from build123d import *

# Parameters (mm, degrees)
F0_R     = 2.25
F0_R_2   = 15.5
F0_R_3   = 13
F1_DEPTH = 15
F2_DEPTH = 3
F3_W     = 12.2
F3_H     = 17.6
F4_DEPTH = 11.3
F5_R     = 1
F6_R     = 3


# Not quite as in the source:
# - ends of sketch curves that miss each other by under 0.0002 mm in the source are joined


with BuildPart() as f1:
    # F0 (on Front) → F1 (new body)
    with BuildSketch(Plane.XZ):
        with BuildLine():
            Line((-0.05, 27.5966813602), (-25.4, 27.5966813602))
            Line((-25.4, 27.5966813602), (-25.4, 7.5966813602))
            Line((-25.4, 7.5966813602), (-21.614542231, 7.5966813602))
            ThreePointArc((-21.614542231, 7.5966813602), (-23.4006244197, -4.2813010605), (-17.918619958, -14.9688724896))
            Line((-17.918619958, -14.9688724896), (-20.4748737342, -17.5251262658))
            ThreePointArc((-20.4748737342, -17.5251262658), (-20.4748737342, -22.4748737342), (-15.5251262658, -22.4748737342))
            Line((-15.5251262658, -22.4748737342), (-13.153804753, -20.1035522213))
            ThreePointArc((-13.153804753, -20.1035522213), (19.3130689129, -14.8757459996), (19.9528476572, 18.0031001889))
            Line((19.9528476572, 18.0031001889), (22.4748737342, 20.5251262658))
            ThreePointArc((22.4748737342, 20.5251262658), (22.4748737342, 25.4748737342), (17.5251262658, 25.4748737342))
            Line((17.5251262658, 25.4748737342), (14.8648475796, 22.8145950479))
            ThreePointArc((14.8648475796, 22.8145950479), (7.8051661925, 26.3642746914), (-9.5e-08, 27.5966326274))
            Line((-9.5e-08, 27.5966326274), (-0.05, 27.5966813602))
        make_face()
        with Locations((-18, -20)):
            Circle(F0_R, mode=Mode.SUBTRACT)
        Circle(F0_R_2, mode=Mode.SUBTRACT)
        with Locations((20, 23)):
            Circle(F0_R, mode=Mode.SUBTRACT)
        Circle(F0_R_2)
        Circle(F0_R_3, mode=Mode.SUBTRACT)
        Circle(F0_R_3)
    extrude(amount=-F1_DEPTH)

    # F0 (on Front) → F2 (cut)
    with BuildSketch(Plane.XZ):
        Circle(F0_R_2)
        Circle(F0_R_3, mode=Mode.SUBTRACT)
    extrude(amount=-F2_DEPTH, mode=Mode.SUBTRACT)

    # F3 (on face) → F4 (cut)
    with BuildSketch(Plane(origin=(-25.4, 0, 0), x_dir=(0, -1, 0), z_dir=(-1, 0, 0))):
        with Locations((-7.1, 17.5966813602)):
            Rectangle(F3_W, F3_H)
    extrude(amount=-F4_DEPTH, mode=Mode.SUBTRACT)

    # F5
    f5_edges = [f1.edges().sort_by_distance(p)[0] for p in [
        (-21.614542, 7.5, 7.596681),
    ]]
    fillet(f5_edges, radius=F5_R)

    # F6
    f6_edges = [f1.edges().sort_by_distance(p)[0] for p in [
        (-17.91862, 7.5, -14.968872),
        (-13.153805, 7.5, -20.103552),
        (19.952848, 7.5, 18.0031),
        (14.864848, 7.5, 22.814595),
    ]]
    fillet(f6_edges, radius=F6_R)


solid = f1.part
Source: CAD feature listing. Evaluate the final solid. Frame: model axes, mm. A direction names the side the tool comes from. Coordinates: 2 decimals unless noted, no trailing zeros. Loops run counter-clockwise (first coordinate to the right, second up) from the corner with the lowest first, then second, coordinate; pieces in that order, holes last. Notation, with made-up numbers: (-21.75, 42) - (19.25, 42) arc R29 cw to (19.25, 72) - close; hole circle Ø7 at (69.25, 68.5). An arc over 180 degrees is marked (long way). One line per item, written item: value. Start each with the question number.
1. Set-up query: faces 1 (the cylindrical face through (6.796, 7.395, 26.666)), 2 (the flat face through (-24, 7, 7.597)), 3 (the cylindrical face through (-16.962, 7.395, -21.996)), 4 (the flat face through (-20, 7, 26.397)), 5 (the cylindrical face through (-2.018, 1.479, 15.368)). Return all of +Z, -Z, +X, -X, +Y, -Y with unobstructed straight access to the full face (end or side cutting, diameter ignored); none if empty.
2. Section A-A (x = 20). Return the cut outline in (y, z).
3. Section D-D (x = 3.5). Return the cut outline in (y, z).
4. Mould query, pull axis Y, two halves, no side actions, for faces 6 (the cylindrical face through (-10.316, 1.479, -7.91)), 7 (the flat face through (-14.1, 7, 18)), 8 (the flat face through (-20, 1, 17)), 9 (the flat face through (3, 3, -13)). Classes: pulls with the +Y half, pulls with the -Y half, needs draft (parallel to the pull), parting line crosses it, or undercut.
5. Ray query, L1, parallel to X at y = 1.5, z = 11.5; L2, parallel to Y at x = -19, z = 10; L3, parallel to Z at x = -20.5, y = 7. Return the intervals inside material, ascending.
6. Contact query for flat-ended pins moving along their axis: P1, Ø1, axis at y = 11, z = 14.5, coming from the -X side; P2, Ø5, axis at y = 5, z = -3, coming from the +X side; P3, Ø9, axis at x = -18.5, y = 4, coming from the -Z side; P4, Ø4, axis at x = 20, z = 23, coming from the +Y side. Output: stop coordinate, or through.
7. Section B-B (y = 4.25). Return the cut outline in (x, z).
8. Section C-C (x = -7.5). Return the cut outline in (y, z), and give its area (3 significant figures).
Verdict:
1. face 1: +Z, +Y, -Y
1. face 2: -X, +Y, -Y
1. face 3: +Y, -Y
1. face 4: -X
1. face 5: -Y
2. outline: (0, -14.05) - (15, -14.05) - (15, 20.75) - (0, 20.75) - close; (0, 25.25) - (15, 25.25) - (15, 26.5) - (0, 26.5) - close
3. outline: (0, -23.46) - (15, -23.46) - (15, 27.35) - (0, 27.35) - (0, 15.1) - (3, 15.1) - (3, 12.52) - (0, 12.52) - (0, -12.52) - (3, -12.52) - (3, -15.1) - (0, -15.1) - close
4. face 6: needs draft
4. face 7: undercut
4. face 8: undercut
4. face 9: pulls with the -Y half
5. L1: x = -14.1 to -10.39, -6.06 to 6.06, 10.39 to 23.75
5. L2: y = 0 to 1, 13.2 to 15
5. L3: z = -22.45 to -17.55, -11.78 to 8.8, 26.4 to 27.6
6. P1: stops at x = -14.1
6. P2: stops at x = 25.48
6. P3: stops at z = -23.5
6. P4: passes through
7. outline: (-25.4, 7.6) - (-23.16, 7.6) arc R1 cw to (-22.23, 6.22) arc R19.59 ccw to (-19.64, -13.01) arc R3 cw to (-19.9, -16.95) - (-20.47, -17.53) arc R3.5 ccw to (-15.53, -22.47) - (-14.73, -21.68) arc R3 cw to (-11.3, -21.11) arc R25.65 ccw to (21.38, 16.04) arc R3 cw to (21.76, 19.81) - (22.47, 20.53) arc R3.5 ccw to (17.53, 25.47) - (16.58, 24.53) arc R3 cw to (12.94, 24.06) arc R25.65 ccw to (0, 27.6) - (-0.05, 27.6) - (-25.4, 27.6) - (-25.4, 26.4) - (-14.1, 26.4) - (-14.1, 8.8) - (-25.4, 8.8) - close; hole circle Ø4.5 at (-18, -20); hole circle Ø4.5 at (20, 23)
8. outline: (0, -22.6) - (15, -22.6) - (15, 27.6) - (0, 27.6) - (0, 13.56) - (3, 13.56) - (3, 10.62) - (0, 10.62) - (0, -10.62) - (3, -10.62) - (3, -13.56) - (0, -13.56) - close
8. area: 735 mm2
